from build123d import *

# Parameters (mm, degrees)
F2_DEPTH      = 25
F2_DEPTH_BACK = 25
F4_DEPTH      = 25
F4_DEPTH_BACK = 25
F6_DEPTH      = 25
F6_DEPTH_BACK = 25


with BuildPart() as f2:
    # F1 (on Front) → F2 (new body, two sides)
    with BuildSketch(Plane.XZ) as f2_sk:
        Polygon((25, 60.3553390593), (-25, 60.3553390593), (-60.3553390593, 25), (-60.3553390593, -25), (-25, -60.3553390593), (25, -60.3553390593), (60.3553390593, -25), (60.3553390593, 25), align=None)
    extrude(amount=F2_DEPTH)
    extrude(f2_sk.sketch, amount=-F2_DEPTH_BACK)

    # F3 (on Top) → F4 (join, two sides)
    with BuildSketch(Plane.XY) as f4_sk:
        Polygon((25, -60.3553390593), (60.3553390593, -25), (60.3553390593, 25), (25, 60.3553390593), (-25, 60.3553390593), (-60.3553390593, 25), (-60.3553390593, -25), (-25, -60.3553390593), align=None)
    extrude(amount=F4_DEPTH)
    extrude(f4_sk.sketch, amount=-F4_DEPTH_BACK)

    # F5 (on Right) → F6 (join, two sides)
    with BuildSketch(Plane.YZ) as f6_sk:
        Polygon((60.3553390593, 25), (25, 60.3553390593), (-25, 60.3553390593), (-60.3553390593, 25), (-60.3553390593, -25), (-25, -60.3553390593), (25, -60.3553390593), (60.3553390593, -25), align=None)
    extrude(amount=F6_DEPTH)
    extrude(f6_sk.sketch, amount=-F6_DEPTH_BACK)


solid = f2.part
Source: CAD feature listing. Evaluate the final solid. Frame: model axes, mm. A direction names the side the tool comes from. Round coordinates to 2 decimals unless told otherwise and drop trailing zeros. Loops run counter-clockwise (first coordinate to the right, second up) from the corner with the lowest first, then second, coordinate; pieces in that order, holes last.
Q1. First-contact query: P1, Ø10.5, axis at x = 48.5, y = 46, coming from the -Z side; P2, Ø17.5, axis at y = 51.5, z = -37, coming from the +X side; P3, Ø17.5, axis at x = 38, y = -46.5, coming from the +Z side; P4, Ø8, axis at y = -19.5, z = -31, coming from the +X side. Flat tips, straight axial feed; report the tip coordinate or a pass-through.
Q2. Section D-D, the plane x = 38.5. Return loops of the section in (y, z).
Q3. Section C-C, the plane y = -29. Return loops of the section in (x, z).
Q4. Ray query, line 1 (X direction, y = -29, z = 52.5); line 2 (Y direction, x = -10, z = -42). Return the intervals inside material, ascending.
Q5. Access query for faces 1 (the face through (39, -39, 25)), 2 (the face through (-35, 35, -25)), 3 (the face through (-35, -35, 25)). Directions: +Z, -Z, +X, -X, +Y, -Y. A direction counts if a zero-diameter tool reaches every point of the face in a straight line with its end or side. Return the directions, or none.
Q6. Section A-A, the plane x = -23. Return loops of the section in (y, z), plus the area to 3 significant figures.
Solutions:
1. P1: passes through
1. P2: stops at x = 25
1. P3: stops at z = 25
1. P4: stops at x = 58.36
2. outline: (-46.86, -25) - (-25, -25) - (-25, -46.86) - (25, -46.86) - (25, -25) - (46.86, -25) - (46.86, 25) - (25, 25) - (25, 46.86) - (-25, 46.86) - (-25, 25) - (-46.86, 25) - close
3. outline: (-56.36, -25) - (-25, -25) - (-25, -56.36) - (25, -56.36) - (25, -25) - (56.36, -25) - (56.36, 25) - (25, 25) - (25, 56.36) - (-25, 56.36) - (-25, 25) - (-56.36, 25) - close
4. line 1: x = -25 to 25
4. line 2: y = -43.36 to 43.36
5. face 1: +Z, +X, -Y
5. face 2: -Z, -X, +Y
5. face 3: +Z, -X, -Y
6. outline: (-60.36, -25) - (-25, -60.36) - (25, -60.36) - (60.36, -25) - (60.36, 25) - (25, 60.36) - (-25, 60.36) - (-60.36, 25) - close
6. area: 12,100 mm2
